Source: CAD feature listing. Evaluate the final solid. Frame: model axes, mm. A direction names the side the tool comes from. Coordinates: 2 decimals unless noted, no trailing zeros. Loops run counter-clockwise (first coordinate to the right, second up) from the corner with the lowest first, then second, coordinate; pieces in that order, holes last. Notation, with made-up numbers: (-26, 85.25) -> (-9, 85.25) arc R17 cw to (-9, 103.25) -> close; hole circle Ø4 at (21.5, 1.25). An arc over 180 degrees is marked (long way). Answer as CSV lines item,"result".
from build123d import *

# Parameters (mm, degrees)
SKETCH_3_W          = 2
SKETCH_3_H          = 2
CUT_EXTRUDE_1_DEPTH = 10


with BuildPart() as part:
    # 草图2 → 旋转1 (revolve)
    with BuildSketch(Plane.XY, mode=Mode.PRIVATE) as revolve_1_sk:
        Polygon((0, 0), (0, 14), (7, 14), (7, 10), (4.5, 10), (4.5, 0), align=None)
    revolve(revolve_1_sk.sketch.rotate(Axis((0, 0, 0), (0, 1, 0)), 90), axis=Axis((0, 0, 0), (0, 1, 0)))

    # 草图3 → 切除-拉伸1 (cut, symmetric)
    with BuildSketch(Plane.XY):
        with Locations((0, 14)):
            Rectangle(SKETCH_3_W, SKETCH_3_H)
    extrude(amount=CUT_EXTRUDE_1_DEPTH, both=True, mode=Mode.SUBTRACT)


solid = part.part
(1) Cut plane C-C (y = 9.5). Return the cut outline in (x, z).
Computed values:
outline,"circle Ø9 at (0, 0)"
(2) Draft query along X for faces 1 (the flat face through (1, 13.5, 0.1)), 2 (the flat face through (-3, 14, 0)), 3 (the cylindrical face through (-3.04, 4.93, 3.32)). Return one class per face: released by +X, released by -X, zero draft, split by the parting line, or undercut.
Computed values:
face 1,"undercut"
face 2,"zero draft"
face 3,"split by the parting line"
(3) Access query for faces 4 (the flat face through (5, 10, 0)), 5 (the flat face through (3, 14, 0)), 6 (the flat face through (0, 13, 0)). Directions: +Z, -Z, +X, -X, +Y, -Y. A direction counts if a zero-diameter tool reaches every point of the face in a straight line with its end or side. Return the directions, or none.
Computed values:
face 4,"-Y"
face 5,"+Z, -Z, +X, -X, +Y"
face 6,"+Z, -Z, +Y"
(4) Material intervals for L1, parallel to Y at x = -1.5, z = 5.75; L2, parallel to Y at x = -0.5, z = -2.5; L3, parallel to X at y = 2.5, z = 0, sorted ascending. Write a range as [from, to].
Computed values:
L1,"[10, 14]"
L2,"[0, 13]"
L3,"[-4.5, 4.5]"
(5) Cut plane D-D (z = -2). Return the cut outline in (x, y), then the cut area to 3 significant figures.
Computed values:
outline,"(-6.71, 10) -> (-4.03, 10) -> (-4.03, 0) -> (4.03, 0) -> (4.03, 10) -> (6.71, 10) -> (6.71, 14) -> (1, 14) -> (1, 13) -> (-1, 13) -> (-1, 14) -> (-6.71, 14) -> close"
area,"132 mm^2"
(6) Pin query (flat end, axial travel): pin 1 Ø1.1 at (y, z) = (13.5, -2) entering from -X; pin 2 Ø2 at (x, z) = (-1.5, -2) entering from -Y; pin 3 Ø1 at (y, z) = (3, -0.5) entering from +X; pin 4 Ø1.1 at (y, z) = (13.5, -2) entering from +X. Return the tip coordinate at first contact, or that it passes through.
Computed values:
pin 1,"x = -6.85"
pin 2,"y = 0"
pin 3,"x = 4.5"
pin 4,"x = 6.85"
(7) Cut plane B-B (x = 0). Return the cut outline in (y, z).
Computed values:
outline,"(0, -4.5) -> (10, -4.5) -> (10, -7) -> (13, -7) -> (13, 7) -> (10, 7) -> (10, 4.5) -> (0, 4.5) -> close"
(8) Cut plane A-A (z = 0). Return the cut outline in (x, y), then the cut area to 3 significant figures.
Computed values:
outline,"(-7, 10) -> (-4.5, 10) -> (-4.5, 0) -> (4.5, 0) -> (4.5, 10) -> (7, 10) -> (7, 14) -> (1, 14) -> (1, 13) -> (-1, 13) -> (-1, 14) -> (-7, 14) -> close"
area,"144 mm^2"
